Build history of the part. All positions in model axes, mm. A direction names the side the tool comes from. Give positions to 0.01 mm unless a question says otherwise; leave off trailing zeros. Answer as CSV lines item,"result".
Autodesk Inventor part; units mm, degrees
ref_plane "YZ Plane" through (0, 0, 0) normal (1, 0, 0) x (0, 1, 0)
ref_plane "XZ Plane" through (0, 0, 0) normal (0, 1, 0) x (-1, 0, 0)
ref_plane "XY Plane" through (0, 0, 0) normal (0, 0, 1) x (1, 0, 0)
sketch "Sketch68" plane through (0, 0, 0) normal (1, 0, 0) x (0, 1, 0)
  line L0 (1, 4.6737) -> (23, 4.6737) construction
  line L1 (7.0021, -2.9903) -> (-7.0029, -0.0135)
  line L2 (7.2385, 26.8729) -> (5.7713, 27.1847)
  line L3 (2.4565, 4.3755) -> (1, 4.6737)
  line L4 (5.7713, 27.1847) -> (1, 4.6737)
  line L5 (7.2385, 26.8729) -> (2.4565, 4.3755)
  point P0 (0, 0)
  point P1 (2.225, 5.1772)
sketch "Sketch184" plane through (0, 0, 0) normal (1, 0, 0) x (0, 1, 0)
  arc A0 (-3.5, -3.0972) -> (0, -1.6204) centre (-4.281, 3.6397) ccw
  arc A1 (0, -1.6204) -> (2.2822, 2) centre (-4.3557, 3.6547) ccw
  arc A2 (2.2822, 2) -> (2.459, 4.3851) centre (-8.8285, 4.0231) ccw
  arc A3 (2.459, 4.3851) -> (2.3883, 6) centre (-72.7121, 1.9029) ccw
  line L0 (-3.5, -3.0972) -> (-3.5, -3.6807)
  arc A4 (2.3883, 6) -> (-3.5, -3.0972) centre (8.6947, -4.5362) ccw
  point P0 (0, 0)
ref_plane "Work Plane13" through (-1.8188, 14.8649, 21.2051) normal (0, 0.8198728, -0.5725457) x (1, 0, 0)
sketch "Sketch199" plane through (-1.8188, 14.8649, 21.2051) normal (0, 0.8198728, -0.5725457) x (1, 0, 0)
  arc A0 (-4.7396, 24.5206) -> (-5.4434, 21.3285) centre (-1.0506, 22.0335) ccw
  arc A1 (-3, 27) -> (-4.7396, 24.5206) centre (12.4104, 14.3381) ccw
  arc A2 (-2.529, 32.2114) -> (-3, 27) centre (13.6873, 28.1188) ccw
  arc A3 (-1.0506, 33.1641) -> (-2.529, 32.2114) centre (-1.0598, 31.555) ccw
  line L0 (-1.0506, 33.1641) -> (5.2457, 33.1641)
  arc A4 (6.5345, 31.555) -> (5.2457, 33.1641) centre (3.9319, 30.7911) ccw
  arc A5 (8.0214, 23.5206) -> (6.5345, 31.555) centre (-50.214, 16.898) ccw
  arc A6 (3.9319, 18.2442) -> (8.0214, 23.5206) centre (2.6688, 23.4462) ccw
  arc A7 (-5.4434, 21.3285) -> (-2.264, 17.7532) centre (-1.0506, 22.0335) ccw
  arc A8 (-2.264, 17.7532) -> (3.9319, 18.2442) centre (-0.0763, 29.4839) ccw
  point P0 (1.8188, 25.8963)
ref_plane "Work Plane14" through (-1.8188, 14.8649, 21.2051) normal (0, 0.8198728, -0.5725457) x (1, 0, 0)
sketch "Sketch200" plane through (-1.8188, 14.8649, 21.2051) normal (0, 0.8198728, -0.5725457) x (1, 0, 0)
  arc A0 (-4.7396, 24.5206) -> (-5.4434, 21.3285) centre (-1.0506, 22.0335) ccw
  arc A1 (-3, 27) -> (-4.7396, 24.5206) centre (12.4104, 14.3381) ccw
  arc A2 (-2.529, 32.2114) -> (-3, 27) centre (13.6873, 28.1188) ccw
  arc A3 (-1.0506, 33.1641) -> (-2.529, 32.2114) centre (-1.0598, 31.555) ccw
  line L0 (-1.0506, 33.1641) -> (5.2457, 33.1641)
  arc A4 (6.5345, 31.555) -> (5.2457, 33.1641) centre (3.9319, 30.7911) ccw
  arc A5 (8.0214, 23.5206) -> (6.5345, 31.555) centre (-50.214, 16.898) ccw
  arc A6 (3.9319, 18.2442) -> (8.0214, 23.5206) centre (2.6688, 23.4462) ccw
  arc A7 (-5.4434, 21.3285) -> (-2.264, 17.7532) centre (-1.0506, 22.0335) ccw
  arc A8 (-2.264, 17.7532) -> (3.9319, 18.2442) centre (-0.0763, 29.4839) ccw
  point P0 (1.8188, 25.8963)
ref_plane "Work Plane15" through (-1.8188, 14.8649, 21.2051) normal (0, 0.8198728, -0.5725457) x (1, 0, 0)
sketch "Sketch201" plane through (-1.8188, 14.8649, 21.2051) normal (0, 0.8198728, -0.5725457) x (1, 0, 0)
  arc A0 (-4.7396, 24.5206) -> (-5.4434, 21.3285) centre (-1.0506, 22.0335) ccw
  arc A1 (-3, 27) -> (-4.7396, 24.5206) centre (12.4104, 14.3381) ccw
  arc A2 (-2.529, 32.2114) -> (-3, 27) centre (13.6873, 28.1188) ccw
  arc A3 (-1.0506, 33.1641) -> (-2.529, 32.2114) centre (-1.0598, 31.555) ccw
  line L0 (-1.0506, 33.1641) -> (5.2457, 33.1641)
  arc A4 (6.5345, 31.555) -> (5.2457, 33.1641) centre (3.9319, 30.7911) ccw
  arc A5 (8.0214, 23.5206) -> (6.5345, 31.555) centre (-50.214, 16.898) ccw
  arc A6 (3.9319, 18.2442) -> (8.0214, 23.5206) centre (2.6688, 23.4462) ccw
  arc A7 (-2.264, 17.7532) -> (3.9319, 18.2442) centre (-0.0763, 29.4839) ccw
  arc A8 (-5.4434, 21.3285) -> (-2.264, 17.7532) centre (-1.0506, 22.0335) ccw
  arc A9 (-4.7396, 24.5206) -> (-5.4434, 21.3285) centre (-1.0506, 22.0335) ccw
  arc A10 (-3, 27) -> (-4.7396, 24.5206) centre (12.4104, 14.3381) ccw
  arc A11 (-2.529, 32.2114) -> (-3, 27) centre (13.6873, 28.1188) ccw
  arc A12 (-1.0506, 33.1641) -> (-2.529, 32.2114) centre (-1.0598, 31.555) ccw
  line L1 (-1.0506, 33.1641) -> (5.2457, 33.1641)
  arc A13 (6.5345, 31.555) -> (5.2457, 33.1641) centre (3.9319, 30.7911) ccw
  arc A14 (8.0214, 23.5206) -> (6.5345, 31.555) centre (-50.214, 16.898) ccw
  arc A15 (3.9319, 18.2442) -> (8.0214, 23.5206) centre (2.6688, 23.4462) ccw
  arc A16 (-2.264, 17.7532) -> (3.9319, 18.2442) centre (-0.0763, 29.4839) ccw
  arc A17 (-5.4434, 21.3285) -> (-2.264, 17.7532) centre (-1.0506, 22.0335) ccw
  arc A18 (-4.7396, 24.5206) -> (-5.4434, 21.3285) centre (-1.0506, 22.0335) ccw
  arc A19 (-3, 27) -> (-4.7396, 24.5206) centre (12.4104, 14.3381) ccw
  arc A20 (-2.529, 32.2114) -> (-3, 27) centre (13.6873, 28.1188) ccw
  arc A21 (-1.0506, 33.1641) -> (-2.529, 32.2114) centre (-1.0598, 31.555) ccw
  line L2 (-1.0506, 33.1641) -> (5.2457, 33.1641)
  arc A22 (6.5345, 31.555) -> (5.2457, 33.1641) centre (3.9319, 30.7911) ccw
  arc A23 (8.0214, 23.5206) -> (6.5345, 31.555) centre (-50.214, 16.898) ccw
  arc A24 (3.9319, 18.2442) -> (8.0214, 23.5206) centre (2.6688, 23.4462) ccw
  arc A25 (-2.264, 17.7532) -> (3.9319, 18.2442) centre (-0.0763, 29.4839) ccw
  arc A26 (-5.4434, 21.3285) -> (-2.264, 17.7532) centre (-1.0506, 22.0335) ccw
  arc A27 (-2.529, 32.2114) -> (-3, 27) centre (13.6873, 28.1188) ccw
  arc A28 (-3, 27) -> (-4.7396, 24.5206) centre (12.4104, 14.3381) ccw
  arc A29 (-4.7396, 24.5206) -> (-5.4434, 21.3285) centre (-1.0506, 22.0335) ccw
  arc A30 (-5.4434, 21.3285) -> (-2.264, 17.7532) centre (-1.0506, 22.0335) ccw
  arc A31 (-2.264, 17.7532) -> (3.9319, 18.2442) centre (-0.0763, 29.4839) ccw
  arc A32 (3.9319, 18.2442) -> (8.0214, 23.5206) centre (2.6688, 23.4462) ccw
  arc A33 (8.0214, 23.5206) -> (6.5345, 31.555) centre (-50.214, 16.898) ccw
  arc A34 (6.5345, 31.555) -> (5.2457, 33.1641) centre (3.9319, 30.7911) ccw
  line L3 (-1.0506, 33.1641) -> (5.2457, 33.1641)
  arc A35 (-1.0506, 33.1641) -> (-2.529, 32.2114) centre (-1.0598, 31.555) ccw
  arc A36 (-3.4348, 34.2537) -> (-4, 28) centre (16.0247, 29.3425) ccw
  arc A37 (-4, 28) -> (-6.0875, 25.0247) centre (14.4925, 12.8057) ccw
  arc A38 (-3.1168, 16.9038) -> (4.3183, 17.4931) centre (-0.4915, 30.9807) ccw
  arc A39 (4.3183, 17.4931) -> (9.2257, 23.8247) centre (2.8025, 23.7355) ccw
  arc A40 (9.2257, 23.8247) -> (7.4414, 33.4659) centre (-60.6567, 15.8776) ccw
  arc A41 (7.4414, 33.4659) -> (5.8948, 35.3969) centre (4.3183, 32.5493) ccw
  line L4 (-1.6607, 35.3969) -> (5.8948, 35.3969)
  arc A42 (-1.6607, 35.3969) -> (-3.4348, 34.2537) centre (-1.6718, 33.4659) ccw
  arc A43 (-6.0875, 25.0247) -> (-6.9321, 21.1943) centre (-1.6607, 22.0403) ccw
  arc A44 (-6.9321, 21.1943) -> (-3.1168, 16.9038) centre (-1.6607, 22.0403) ccw
  point P0 (1.8188, 25.8963)
sketch "Sketch213" plane through (0, 0, 0) normal (1, 0, 0) x (0, 1, 0)
  line L0 (13.3414, -11.8728) -> (-10.8201, 5)
  line L1 (46.9769, 13.1952) -> (16.4024, 18.5466)
  line L2 (-15.4661, -26.0463) -> (-0.3893, -51.1005)
  line L3 (-0.3893, -51.1005) -> (1.9473, -49.7476)
  line L4 (46.9769, 13.1952) -> (46.7355, 11.8161)
  line L5 (1.9473, -49.7476) -> (-11.7207, -26.1425)
  line L6 (-11.7207, -26.1425) -> (-10, -24)
  line L7 (-10, -24) -> (-10.853, -23.4043)
  line L8 (46.7355, 11.8161) -> (18.2275, 16.8059)
  line L9 (18.2275, 16.8059) -> (17, 15)
  line L10 (17, 15) -> (16.3637, 15.4444)
  line L11 (16.3637, 15.4444) -> (17.062, 16.4444)
  line L12 (17.062, 16.4444) -> (17.3561, 17.7094)
  line L13 (17.3561, 17.7094) -> (16.3637, 17.6698)
  line L14 (16.3637, 17.6698) -> (16.4024, 18.5466)
  line L15 (-10.853, -23.4043) -> (-11.9333, -25.0763)
  line L16 (-11.9333, -25.0763) -> (-13.146, -25.8811)
  line L17 (-13.146, -25.8811) -> (-12.9536, -24.5344)
  line L18 (-12.9536, -24.5344) -> (-15.4661, -26.0463)
  point P0 (0, 0)
  point P1 (3.3399, -2.2736)
  point P2 (-1.2043, -8.7808)
  dimension "d600" = 2.7
  dimension "d601" = 1.4
  dimension "d603" = 1.265
revolve "Revolution6" add sketch "Sketch213" angle 180 mid plane about axis through (0, 13.3414, -11.8728) along (0, -0.8198728, 0.5725457) contours L18 L17 L16 L15 L7 L6 L5 L3 L2
sketch "Sketch214" plane through (-28.1141, 0.6305, -2.9963) normal (0, 0.5725457, 0.8198728) x (0.9133048, 0.3339151, -0.2331846)
  line L0 (71.2508, -4.0445) -> (70.3985, -3.0629)
  line L1 (70.3985, -3.0629) -> (64.3578, -8.3078)
  line L2 (71.2508, -4.0445) -> (65.2101, -9.2894)
  line L3 (64.3578, -8.3078) -> (65.2101, -9.2894)
  line L4 (2.6996, 29.2863) -> (0, 29.2408)
  line L5 (3.1595, 2.0136) -> (2.6996, 29.2863)
  line L6 (0, 29.2408) -> (0, 0)
  line L7 (0.7, 27.3772) -> (2, 27.3772)
  line L8 (0.7, 27.3772) -> (0.7, 19.3772)
  line L9 (2, 27.3772) -> (2, 19.3772)
  line L10 (0.7, 19.3772) -> (2, 19.3772)
  line L11 (51.3534, -22.9004) -> (73.1067, -3.3602)
  line L12 (73.1067, -3.3602) -> (71.3365, -1.3215)
  line L13 (71.3365, -1.3215) -> (50.7401, -19.2043)
  point P0 (24.7675, -13.4891)
  dimension "d606" = 8
  dimension "d625" = 90
  dimension "d626" = 0.7
  dimension "d630" = 1.3
  dimension "d635" = 0.7
  dimension "d637" = 1.85
extrude "Extrusion162" add sketch "Sketch214" along normal blind 3
properties part number "A1_V1_M2_dropArm_WOK_meso_tall_VIS_rt"
Item 1: Pull direction Z, two halves, no side cores. Call faces 4 (the cylindrical face through (-0.513, -10.429, -23.693)), 5 (the conical face through (0.564, -12.983, -24.763)), 6 (the conical face through (0.69, -11.17, -33.17)): released by +Z, released by -Z, zero draft, split by the parting line, or undercut.
Geometry says:
face 4,"released by +Z"
face 5,"undercut"
face 6,"split by the parting line"
Item 2: Drop flat-ended pins along their axis: pin 1 (1.5 mm diameter, centred on y = 1, z = -25, fed in from +X); pin 2 (2 mm diameter, centred on x = 31, z = -31, fed in from -Y); pin 3 (1.5 mm diameter, centred on x = 19.5, z = -26, fed in from -Y). Give the stop position or say it passes through.
Geometry says:
pin 1,"stops at x = 29.39"
pin 2,"stops at y = 4.16"
pin 3,"stops at y = -8.76"
Item 3: Probe line 1 along X through (y, z) = (-7, -24); line 2 along X through (y, z) = (1.5, -39); line 3 along Y through (x, z) = (-17, -39). List the from-to ranges inside material, lowest first. Write a range as from..to.
Geometry says:
line 1,"x = -21.81..-16.68, 16.68..21.81"
line 2,"x = -23.95..-18.72, 18.72..23.95"
line 3,"y = -3.11..0.47"
Item 4: 3-axis set-ups, long thin cutter, end or side, ignore diameter. For faces 1 (the conical face through (0.52, -11.037, -23.69)), 2 (the flat face through (-37.02, 19.26, -14.2)), 3 (the flat face through (38.03, 22.46, -16.44)): which of +Z, -Z, +X, -X, +Y, -Y reach the whole face in a straight line?
Geometry says:
face 1,"+Z"
face 2,"+Z, -X"
face 3,"+X, +Y"
